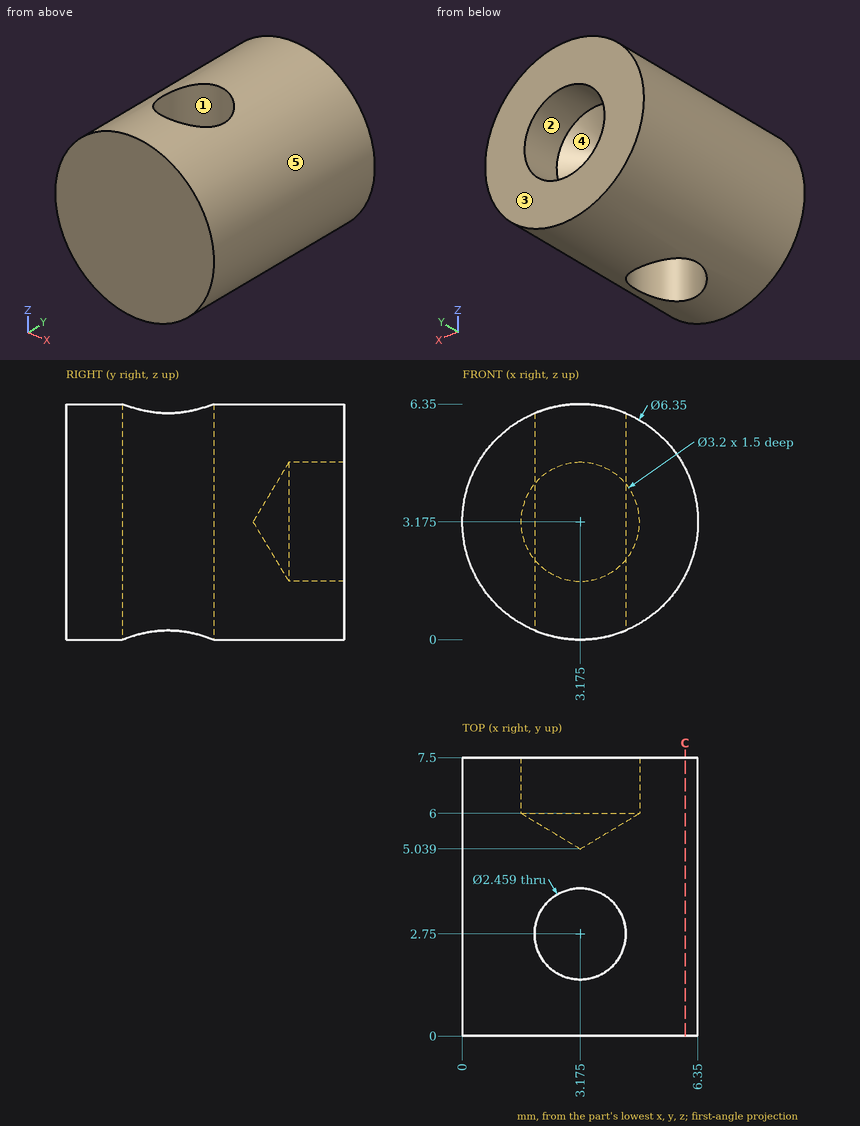
Verification items for this drawing (mm, ordinates from the low corner). A direction names the side the tool comes from. Coordinates: 2 decimals unless noted, no trailing zeros. Write each loop counter-clockwise with the first axis right and the second up, starting at its lowest first coordinate (ties: lowest second). Pieces come first, ordered by that corner, then holes. Notation, with made-up numbers: M 74.25,50.5 L 97.25,50.5 A26 cw 97.25,83.5 Z; hole C 70,66.25 d8. An arc over 180 degrees is marked long. Answer as a JSON object with one key per item and string values.
1. Go/stop test with flat-tipped pins: pin 1 Ø2 at (x, z) = (2.5, 4) entering from +Y; pin 2 Ø1.9 at (x, z) = (3.175, 3.175) entering from +Y; pin 3 Ø1.5 at (x, y) = (5, 6) entering from +Z. Record where each tip stops, or that it passes through.
Answers below:
{"pin 1": "stops at y = 7.5", "pin 2": "stops at y = 5.61", "pin 3": "stops at z = 6.16"}
2. Scan lines: L1, parallel to X at y = 7, z = 3 (1 decimal); L2, parallel to X at y = 2.75, z = 3.5 (1 decimal); L3, parallel to Y at x = 2.5, z = 3.75. Record each from-to range of solid material in increasing order.
Answers below:
{"L1": "x = 0 to 1.6, 4.8 to 6.3", "L2": "x = 0 to 1.9, 4.4 to 6.3", "L3": "y = 0 to 1.72, 3.78 to 5.57"}
3. Section check C-C, the plane x = 6. Enter the section's corners in (y, z) (1 decimal).
Answers below:
{"outline": "M 0,1.7 L 7.5,1.7 L 7.5,4.6 L 0,4.6 Z"}
4. Draft check along X on the marked faces 3, 4 and 5. Enter one of: released by +X, released by -X, zero draft, split by the parting line, or undercut.
Answers below:
{"face 3": "zero draft", "face 4": "undercut", "face 5": "split by the parting line"}
5. Tool access check on the marked faces 1 and 2. Record the directions out of +Z, -Z, +X, -X, +Y, -Y that give a thin tool (end or side, any length) a straight path to the whole face; none if there is none.
Answers below:
{"face 1": "+Z, -Z", "face 2": "+Y"}
